Autodesk Inventor part; units mm, degrees
ref_plane "YZ Plane" through (0, 0, 0) normal (1, 0, 0) x (0, 1, 0)
ref_plane "XZ Plane" through (0, 0, 0) normal (0, 1, 0) x (-1, 0, 0)
ref_plane "XY Plane" through (0, 0, 0) normal (0, 0, 1) x (1, 0, 0)
sketch "Esboço2" plane through (0, 0, 0) normal (0, 0, 1) x (1, 0, 0)
  line L0 (0, 0) -> (9.5, 0)
  line L1 (9.5, 0) -> (9.5, 9.8)
  line L2 (9.5, 9.8) -> (0, 9.8)
  line L3 (0, 9.8) -> (0, 0)
  line L4 (9.5, 0) -> (1, 0)
  line L5 (9.5, 0) -> (0.5, 0)
  line L6 (0, 0) -> (1, 0)
  line L7 (1, 0) -> (1, 9.8)
  dimension "d0" = 9.5
  dimension "d1" = 9.8
  dimension "d71" = 8.5
  dimension "d72" = 9
revolve "Revolução1" add sketch "Esboço2" angle 360 about axis through (0, 0, 0) along (1, 0, 0) contours L7 L2 L1 L0
sketch "Esboço12" plane through (9.5, 0, 0) normal (1, 0, 0) x (0, 0, -1)
  point P0 (0, 0)
sketch "Esboço13" plane through (1, 0, 0) normal (-1, 0, 0) x (0, 0, 1)
  circle A0 centre (0, 0) radius 1.75
  dimension "d73" = 3.5
extrude "Extrusão6" cut sketch "Esboço13" against normal blind 3.85
sketch "Esboço14" plane through (1, 0, 0) normal (-1, 0, 0) x (0, 0, 1)
  circle A0 centre (0, 0) radius 1.75
  circle A1 centre (0, 0) radius 4.5
  dimension "d76" = 9
extrude "Extrusão7" cut sketch "Esboço14" against normal blind 1
sketch "Esboço15" plane through (9.5, 0, 0) normal (1, 0, 0) x (0, 0, -1)
  circle A0 centre (0, 0) radius 2.5
  circle A1 centre (0, 0) radius 1.75
  circle A2 centre (0, 0) radius 2.9
  line L0 (2.5, 0) -> (2.5, 0.05)
  line L1 (2.5, 0) -> (2.4995, -0.05)
  line L2 (2.4995, -0.05) -> (2.8824, -0.3191)
  line L3 (2.5, 0.05) -> (2.8824, 0.3191)
  line L4 (2.8824, 0.3191) -> (2.8765, 0.3688)
  line L5 (2.8824, -0.3191) -> (2.8824, -0.3191)
  line L6 (2.8824, -0.3191) -> (2.8824, -0.3191)
  line L7 (2.8824, -0.3191) -> (2.8824, -0.3191)
  line L8 (2.8824, -0.3191) -> (2.8824, -0.3191)
  line L9 (2.8824, -0.3191) -> (2.8824, -0.3191)
  line L10 (2.8795, -0.3439) -> (2.8795, -0.3439)
  line L11 (2.8824, -0.3191) -> (2.8824, -0.3191)
  line L12 (2.3622, 0.8201) -> (2.6427, 1.1942)
  line L13 (2.6427, 1.1942) -> (2.6217, 1.2396)
  line L14 (2.3776, 0.7725) -> (2.3622, 0.8201)
  line L15 (2.3776, 0.7725) -> (2.3926, 0.7248)
  line L16 (2.3926, 0.7248) -> (2.8399, 0.5872)
  circle A3 centre (0, 0) radius 2.9
  line L17 (1.9932, 1.5099) -> (2.1443, 1.9524)
  line L18 (2.1443, 1.9524) -> (2.1104, 1.9891)
  line L19 (2.0225, 1.4695) -> (1.9932, 1.5099)
  line L20 (2.0225, 1.4695) -> (2.0515, 1.4287)
  line L21 (2.0515, 1.4287) -> (2.5195, 1.4361)
  circle A4 centre (0, 0) radius 2.9
  line L22 (1.429, 2.0519) -> (1.4361, 2.5195)
  line L23 (1.4361, 2.5195) -> (1.3924, 2.5439)
  line L24 (1.4695, 2.0225) -> (1.429, 2.0519)
  line L25 (1.4695, 2.0225) -> (1.5096, 1.9928)
  line L26 (1.5096, 1.9928) -> (1.9524, 2.1443)
  circle A5 centre (0, 0) radius 2.9
  line L27 (0.725, 2.3931) -> (0.5872, 2.8399)
  line L28 (0.5872, 2.8399) -> (0.5382, 2.8496)
  line L29 (0.7725, 2.3776) -> (0.725, 2.3931)
  line L30 (0.7725, 2.3776) -> (0.8199, 2.3617)
  line L31 (0.8199, 2.3617) -> (1.1942, 2.6427)
  circle A6 centre (0, 0) radius 2.9
  line L32 (-0.05, 2.5) -> (-0.3191, 2.8824)
  line L33 (-0.3191, 2.8824) -> (-0.3688, 2.8765)
  line L34 (0, 2.5) -> (-0.05, 2.5)
  line L35 (0, 2.5) -> (0.05, 2.4995)
  line L36 (0.05, 2.4995) -> (0.3191, 2.8824)
  circle A7 centre (0, 0) radius 2.9
  line L37 (-0.8201, 2.3622) -> (-1.1942, 2.6427)
  line L38 (-1.1942, 2.6427) -> (-1.2396, 2.6217)
  line L39 (-0.7725, 2.3776) -> (-0.8201, 2.3622)
  line L40 (-0.7725, 2.3776) -> (-0.7248, 2.3926)
  line L41 (-0.7248, 2.3926) -> (-0.5872, 2.8399)
  circle A8 centre (0, 0) radius 2.9
  line L42 (-1.5099, 1.9932) -> (-1.9524, 2.1443)
  line L43 (-1.9524, 2.1443) -> (-1.9891, 2.1104)
  line L44 (-1.4695, 2.0225) -> (-1.5099, 1.9932)
  line L45 (-1.4695, 2.0225) -> (-1.4287, 2.0515)
  line L46 (-1.4287, 2.0515) -> (-1.4361, 2.5195)
  circle A9 centre (0, 0) radius 2.9
  line L47 (-2.0519, 1.429) -> (-2.5195, 1.4361)
  line L48 (-2.5195, 1.4361) -> (-2.5439, 1.3924)
  line L49 (-2.0225, 1.4695) -> (-2.0519, 1.429)
  line L50 (-2.0225, 1.4695) -> (-1.9928, 1.5096)
  line L51 (-1.9928, 1.5096) -> (-2.1443, 1.9524)
  circle A10 centre (0, 0) radius 2.9
  line L52 (-2.3931, 0.725) -> (-2.8399, 0.5872)
  line L53 (-2.8399, 0.5872) -> (-2.8496, 0.5382)
  line L54 (-2.3776, 0.7725) -> (-2.3931, 0.725)
  line L55 (-2.3776, 0.7725) -> (-2.3617, 0.8199)
  line L56 (-2.3617, 0.8199) -> (-2.6427, 1.1942)
  circle A11 centre (0, 0) radius 2.9
  line L57 (-2.5, -0.05) -> (-2.8824, -0.3191)
  line L58 (-2.8824, -0.3191) -> (-2.8765, -0.3688)
  line L59 (-2.5, 0) -> (-2.5, -0.05)
  line L60 (-2.5, 0) -> (-2.4995, 0.05)
  line L61 (-2.4995, 0.05) -> (-2.8824, 0.3191)
  circle A12 centre (0, 0) radius 2.9
  line L62 (-2.3622, -0.8201) -> (-2.6427, -1.1942)
  line L63 (-2.6427, -1.1942) -> (-2.6217, -1.2396)
  line L64 (-2.3776, -0.7725) -> (-2.3622, -0.8201)
  line L65 (-2.3776, -0.7725) -> (-2.3926, -0.7248)
  line L66 (-2.3926, -0.7248) -> (-2.8399, -0.5872)
  circle A13 centre (0, 0) radius 2.9
  line L67 (-1.9932, -1.5099) -> (-2.1443, -1.9524)
  line L68 (-2.1443, -1.9524) -> (-2.1104, -1.9891)
  line L69 (-2.0225, -1.4695) -> (-1.9932, -1.5099)
  line L70 (-2.0225, -1.4695) -> (-2.0515, -1.4287)
  line L71 (-2.0515, -1.4287) -> (-2.5195, -1.4361)
  circle A14 centre (0, 0) radius 2.9
  line L72 (-1.429, -2.0519) -> (-1.4361, -2.5195)
  line L73 (-1.4361, -2.5195) -> (-1.3924, -2.5439)
  line L74 (-1.4695, -2.0225) -> (-1.429, -2.0519)
  line L75 (-1.4695, -2.0225) -> (-1.5096, -1.9928)
  line L76 (-1.5096, -1.9928) -> (-1.9524, -2.1443)
  circle A15 centre (0, 0) radius 2.9
  line L77 (-0.725, -2.3931) -> (-0.5872, -2.8399)
  line L78 (-0.5872, -2.8399) -> (-0.5382, -2.8496)
  line L79 (-0.7725, -2.3776) -> (-0.725, -2.3931)
  line L80 (-0.7725, -2.3776) -> (-0.8199, -2.3617)
  line L81 (-0.8199, -2.3617) -> (-1.1942, -2.6427)
  circle A16 centre (0, 0) radius 2.9
  line L82 (0.05, -2.5) -> (0.3191, -2.8824)
  line L83 (0.3191, -2.8824) -> (0.3688, -2.8765)
  line L84 (0, -2.5) -> (0.05, -2.5)
  line L85 (0, -2.5) -> (-0.05, -2.4995)
  line L86 (-0.05, -2.4995) -> (-0.3191, -2.8824)
  circle A17 centre (0, 0) radius 2.9
  line L87 (0.8201, -2.3622) -> (1.1942, -2.6427)
  line L88 (1.1942, -2.6427) -> (1.2396, -2.6217)
  line L89 (0.7725, -2.3776) -> (0.8201, -2.3622)
  line L90 (0.7725, -2.3776) -> (0.7248, -2.3926)
  line L91 (0.7248, -2.3926) -> (0.5872, -2.8399)
  circle A18 centre (0, 0) radius 2.9
  line L92 (1.5099, -1.9932) -> (1.9524, -2.1443)
  line L93 (1.9524, -2.1443) -> (1.9891, -2.1104)
  line L94 (1.4695, -2.0225) -> (1.5099, -1.9932)
  line L95 (1.4695, -2.0225) -> (1.4287, -2.0515)
  line L96 (1.4287, -2.0515) -> (1.4361, -2.5195)
  circle A19 centre (0, 0) radius 2.9
  line L97 (2.0519, -1.429) -> (2.5195, -1.4361)
  line L98 (2.5195, -1.4361) -> (2.5439, -1.3924)
  line L99 (2.0225, -1.4695) -> (2.0519, -1.429)
  line L100 (2.0225, -1.4695) -> (1.9928, -1.5096)
  line L101 (1.9928, -1.5096) -> (2.1443, -1.9524)
  circle A20 centre (0, 0) radius 2.9
  line L102 (2.3931, -0.725) -> (2.8399, -0.5872)
  line L103 (2.8399, -0.5872) -> (2.8496, -0.5382)
  line L104 (2.3776, -0.7725) -> (2.3931, -0.725)
  line L105 (2.3776, -0.7725) -> (2.3617, -0.8199)
  line L106 (2.3617, -0.8199) -> (2.6427, -1.1942)
  circle A21 centre (0, 0) radius 2.9
  point P0 (2.8399, 0.5872)
  point P1 (2.8399, 0.5872)
  point P2 (2.8399, 0.5872)
  point P3 (2.8399, 0.5872)
  point P4 (2.8399, 0.5872)
  point P5 (2.8449, 0.5627)
  point P6 (2.8449, 0.5627)
  point P7 (2.8399, 0.5872)
  point P8 (2.5195, 1.4361)
  point P9 (2.5195, 1.4361)
  point P10 (2.5195, 1.4361)
  point P11 (2.5195, 1.4361)
  point P12 (2.5195, 1.4361)
  point P13 (2.5318, 1.4143)
  point P14 (2.5318, 1.4143)
  point P15 (2.5195, 1.4361)
  point P16 (1.9524, 2.1443)
  point P17 (1.9524, 2.1443)
  point P18 (1.9524, 2.1443)
  point P19 (1.9524, 2.1443)
  point P20 (1.9524, 2.1443)
  point P21 (1.9708, 2.1274)
  point P22 (1.9708, 2.1274)
  point P23 (1.9524, 2.1443)
  point P24 (1.1942, 2.6427)
  point P25 (1.1942, 2.6427)
  point P26 (1.1942, 2.6427)
  point P27 (1.1942, 2.6427)
  point P28 (1.1942, 2.6427)
  point P29 (1.2169, 2.6323)
  point P30 (1.2169, 2.6323)
  point P31 (1.1942, 2.6427)
  point P32 (0.3191, 2.8824)
  point P33 (0.3191, 2.8824)
  point P34 (0.3191, 2.8824)
  point P35 (0.3191, 2.8824)
  point P36 (0.3191, 2.8824)
  point P37 (0.3439, 2.8795)
  point P38 (0.3439, 2.8795)
  point P39 (0.3191, 2.8824)
  point P40 (-0.5872, 2.8399)
  point P41 (-0.5872, 2.8399)
  point P42 (-0.5872, 2.8399)
  point P43 (-0.5872, 2.8399)
  point P44 (-0.5872, 2.8399)
  point P45 (-0.5627, 2.8449)
  point P46 (-0.5627, 2.8449)
  point P47 (-0.5872, 2.8399)
  point P48 (-1.4361, 2.5195)
  point P49 (-1.4361, 2.5195)
  point P50 (-1.4361, 2.5195)
  point P51 (-1.4361, 2.5195)
  point P52 (-1.4361, 2.5195)
  point P53 (-1.4143, 2.5318)
  point P54 (-1.4143, 2.5318)
  point P55 (-1.4361, 2.5195)
  point P56 (-2.1443, 1.9524)
  point P57 (-2.1443, 1.9524)
  point P58 (-2.1443, 1.9524)
  point P59 (-2.1443, 1.9524)
  point P60 (-2.1443, 1.9524)
  point P61 (-2.1274, 1.9708)
  point P62 (-2.1274, 1.9708)
  point P63 (-2.1443, 1.9524)
  point P64 (-2.6427, 1.1942)
  point P65 (-2.6427, 1.1942)
  point P66 (-2.6427, 1.1942)
  point P67 (-2.6427, 1.1942)
  point P68 (-2.6427, 1.1942)
  point P69 (-2.6323, 1.2169)
  point P70 (-2.6323, 1.2169)
  point P71 (-2.6427, 1.1942)
  point P72 (-2.8824, 0.3191)
  point P73 (-2.8824, 0.3191)
  point P74 (-2.8824, 0.3191)
  point P75 (-2.8824, 0.3191)
  point P76 (-2.8824, 0.3191)
  point P77 (-2.8795, 0.3439)
  point P78 (-2.8795, 0.3439)
  point P79 (-2.8824, 0.3191)
  point P80 (-2.8399, -0.5872)
  point P81 (-2.8399, -0.5872)
  point P82 (-2.8399, -0.5872)
  point P83 (-2.8399, -0.5872)
  point P84 (-2.8399, -0.5872)
  point P85 (-2.8449, -0.5627)
  point P86 (-2.8449, -0.5627)
  point P87 (-2.8399, -0.5872)
  point P88 (-2.5195, -1.4361)
  point P89 (-2.5195, -1.4361)
  point P90 (-2.5195, -1.4361)
  point P91 (-2.5195, -1.4361)
  point P92 (-2.5195, -1.4361)
  point P93 (-2.5318, -1.4143)
  point P94 (-2.5318, -1.4143)
  point P95 (-2.5195, -1.4361)
  point P96 (-1.9524, -2.1443)
  point P97 (-1.9524, -2.1443)
  point P98 (-1.9524, -2.1443)
  point P99 (-1.9524, -2.1443)
  point P100 (-1.9524, -2.1443)
  point P101 (-1.9708, -2.1274)
  point P102 (-1.9708, -2.1274)
  point P103 (-1.9524, -2.1443)
  point P104 (-1.1942, -2.6427)
  point P105 (-1.1942, -2.6427)
  point P106 (-1.1942, -2.6427)
  point P107 (-1.1942, -2.6427)
  point P108 (-1.1942, -2.6427)
  point P109 (-1.2169, -2.6323)
  point P110 (-1.2169, -2.6323)
  point P111 (-1.1942, -2.6427)
  point P112 (-0.3191, -2.8824)
  point P113 (-0.3191, -2.8824)
  point P114 (-0.3191, -2.8824)
  point P115 (-0.3191, -2.8824)
  point P116 (-0.3191, -2.8824)
  point P117 (-0.3439, -2.8795)
  point P118 (-0.3439, -2.8795)
  point P119 (-0.3191, -2.8824)
  point P120 (0.5872, -2.8399)
  point P121 (0.5872, -2.8399)
  point P122 (0.5872, -2.8399)
  point P123 (0.5872, -2.8399)
  point P124 (0.5872, -2.8399)
  point P125 (0.5627, -2.8449)
  point P126 (0.5627, -2.8449)
  point P127 (0.5872, -2.8399)
  point P128 (1.4361, -2.5195)
  point P129 (1.4361, -2.5195)
  point P130 (1.4361, -2.5195)
  point P131 (1.4361, -2.5195)
  point P132 (1.4361, -2.5195)
  point P133 (1.4143, -2.5318)
  point P134 (1.4143, -2.5318)
  point P135 (1.4361, -2.5195)
  point P136 (2.1443, -1.9524)
  point P137 (2.1443, -1.9524)
  point P138 (2.1443, -1.9524)
  point P139 (2.1443, -1.9524)
  point P140 (2.1443, -1.9524)
  point P141 (2.1274, -1.9708)
  point P142 (2.1274, -1.9708)
  point P143 (2.1443, -1.9524)
  point P144 (2.6427, -1.1942)
  point P145 (2.6427, -1.1942)
  point P146 (2.6427, -1.1942)
  point P147 (2.6427, -1.1942)
  point P148 (2.6427, -1.1942)
  point P149 (2.6323, -1.2169)
  point P150 (2.6323, -1.2169)
  point P151 (2.6427, -1.1942)
  dimension "d79" = 5
  dimension "d80" = 5.8
  dimension "d81" = 0.05
  dimension "d82" = 0.05
  dimension "d83" = 0.468
  dimension "d85" = 0.05
  dimension "d88" = 360
extrude "Extrusão8" cut sketch "Esboço15" against normal blind 3.5 contours A0 | A0 L16 A2 L3 | L2 A2 L102 A0 | A0 L21 A2 L12 | L106 A2 L97 A0 | A0 L26 A2 L17 | L101 A2 L92 A0 | A0 L31 A2 L22 | L96 A2 L87 A0 | A0 L36 A2 L27 | L91 A2 L82 A0 | A0 L41 A2 L32 | L86 A2 L77 A0 | A0 L46 A2 L37 | L81 A2 L72 A0 | A0 L51 A2 L42 | L76 A2 L67 A0 | A0 L56 A2 L47 | L71 A2 L62 A0 | A0 L61 A2 L52 | L66 A2 L57 A0 | A1
properties part number "roda certa 3.0"
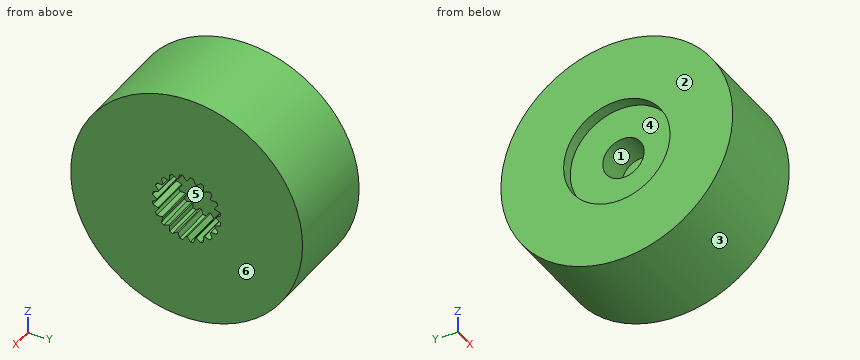
Work out the finished part from the listing and answer in its coordinate system (mm). Face numbers are marked on the shaded views. A direction names the side the tool comes from. Round coordinates to 2 decimals unless told otherwise and drop trailing zeros. Write each loop counter-clockwise with the first axis right and the second up, starting at its lowest first coordinate (ties: lowest second). Pieces come first, ordered by that corner, then holes. Notation, with made-up numbers: (10.5, -1.5) -> (36.5, -1.5) arc R26 cw to (36.5, 31.5) -> close; hole circle Ø3 at (82, -18). An arc over 180 degrees is marked (long way). Write each question's results on one line, items separated by ' | '.
Item 1: A cutting plane is placed at A-A, the plane x = 3.25. Determine the outline of the cut face in (y, z).
Result set:
outline: circle Ø19.6 at (0, 0); hole circle Ø3.5 at (0, 0)
Item 2: Which of the six approach directions +Z, -Z, +X, -X, +Y, -Y give full straight-line access (tool end or side, diameter ignored) to the marked faces 4, 5 and 6?
Result set:
face 4: -X | face 5: +X | face 6: +Z, -Z, +X, +Y, -Y
Item 3: Find the intervals of material crossed by line 1 along X through (y, z) = (0.25, -1.5); line 2 along X through (y, z) = (-2.75, 0); line 3 along Z through (x, y) = (8.75, 0.25), in increasing order. Write a range as [from, to].
Result set:
line 1: [4.85, 6] | line 2: [2, 9.5] | line 3: [-9.8, -2.78], [2.78, 9.8]
Item 4: The mould has two halves that part along Y. Classify the marked faces 1, 2 and 3: +Y half, -Y half, draft (parallel to the pull), parting line (faces both ways), or undercut.
Result set:
face 1: undercut | face 2: draft | face 3: parting line
Item 5: A cutting plane is placed at C-C, the plane y = -5.75. Determine the outline of the cut face in (x, z), plus the area to 3 significant figures.
Result set:
outline: (1, -7.94) -> (9.5, -7.94) -> (9.5, 7.94) -> (1, 7.94) -> close | area: 135 mm^2
Item 6: A cutting plane is placed at B-B, the plane z = -7.5. Determine the outline of the cut face in (x, y).
Result set:
outline: (1, -6.31) -> (9.5, -6.31) -> (9.5, 6.31) -> (1, 6.31) -> close
Item 7: Flat-ended cylindrical pins translate along their axes: P1, Ø1.5, axis at x = 4.5, y = -7, coming from the +Z side; P2, Ø3, axis at x = 7, z = 3, coming from the +Y side; P3, Ø3, axis at y = 0, z = 0, coming from the -X side. Find the tip coordinate at first contact, or state that the pin passes through.
Result set:
P1: z = 7.55 | P2: y = 9.68 | P3: x = 4.85
